CAD build for the part. Positions are in the model's coordinates, mm. A direction names the side the tool comes from. Give positions to 0.01 mm unless a question says otherwise; leave off trailing zeros. Write each loop counter-clockwise with the first axis right and the second up, starting at its lowest first coordinate (ties: lowest second). Pieces come first, ordered by that corner, then holes. Notation, with made-up numbers: (-30, 8) - (16, 8) arc R29 ccw to (16, 35) - close; hole circle Ø6 at (-3, 13). An arc over 180 degrees is marked (long way). Put each result on its own line as item: value. Start each with the question number.
1. Mould opens along X. For faces 3 (the cylindrical face through (0.16, 21.937, 5.916)), 4 (the cylindrical face through (-10.28, -7.77, 0.85)), 5 (the flat face through (0, 0, -10)) say: +X half, -X half, draft (parallel to the pull), parting line (faces both ways), or undercut.
2. Tool access for faces 1 (the flat face through (-1, 1, 12)), 2 (the cylindrical face through (-0.618, 57.997, 5.916)): list every direction of +Z, -Z, +X, -X, +Y, -Y with a clear straight run to the whole face (end or side of a thin tool).
3. Cut at D-D on x = 33.5. List the corners of the cut face in (y, z), and give its area (3 significant figures).
4. Cut at B-B on z = 9.25. Give the number of separate pieces and of enclosed holes in the cut face, and give its area (3 significant figures).
5. Cut at A-A on y = -14. List the corners of the cut face in (x, z).
6. Drop flat-ended pins along their axis: pin 1 (10 mm diameter, centred on y = -51.5, z = -2.5, fed in from -X); pin 2 (3 mm diameter, centred on y = 54, z = 4.5, fed in from +X); pin 3 (3.5 mm diameter, centred on x = -12.12, y = 7, fed in from -Z); pin 4 (5 mm diameter, centred on x = 60, z = 6, fed in from -Y). Give the stop position or say it passes through.
7. Wall check: line 1 (Y direction, x = 0, z = -1.75); line 2 (Y direction, x = 0, z = 6.5); line 3 (Y direction, x = 25, z = 1.25). Give the ranges that are in metal, low to high.
8. Cut at C-C on y = 7. List the corners of the cut face in (x, z), and give its area (3 significant figures).
from build123d import *

# Parameters (mm, degrees)
SKETCH1_R               = 85
SKETCH1_R_2             = 2
BOSS_EXTRUDE1_DEPTH     = 12
SKETCH3_R               = 22
BOSS_EXTRUDE2_DEPTH     = 10
CUT_EXTRUDE1_DEPTH      = 123.204746225
CUT_EXTRUDE1_DEPTH_BACK = 123.204746225
SKETCH5_R               = 2


with BuildPart() as part:
    # Sketch1 → Boss-Extrude1 (new body)
    with BuildSketch(Plane.XY):
        Circle(SKETCH1_R)
        with Locations((0, 14)):
            Circle(SKETCH1_R_2, mode=Mode.SUBTRACT)
        with Locations((12.124355653, 7)):
            Circle(SKETCH1_R_2, mode=Mode.SUBTRACT)
        with Locations((12.124355653, -7)):
            Circle(SKETCH1_R_2, mode=Mode.SUBTRACT)
        with Locations((0, -14)):
            Circle(SKETCH1_R_2, mode=Mode.SUBTRACT)
        with Locations((-12.124355653, -7)):
            Circle(SKETCH1_R_2, mode=Mode.SUBTRACT)
        with Locations((-12.124355653, 7)):
            Circle(SKETCH1_R_2, mode=Mode.SUBTRACT)
        with BuildLine():
            Line((-16.104768385, 19.179115852), (-39.269994022, 34.182407181))
            ThreePointArc((-39.269994022, 34.182407181), (-41.530272968, 37.914054118), (-40.000243417, 41.999768173))
            ThreePointArc((-40.000243417, 41.999768173), (0, 58), (40.000243417, 41.999768173))
            ThreePointArc((40.000243417, 41.999768173), (41.530272968, 37.914054118), (39.269994022, 34.182407181))
            Line((39.269994022, 34.182407181), (16.104768385, 19.179115852))
            ThreePointArc((16.104768385, 19.179115852), (13.523321314, 18.377673488), (10.90195317, 19.036921468))
            ThreePointArc((10.90195317, 19.036921468), (0, 21.937569645), (-10.90195317, 19.036921468))
            ThreePointArc((-10.90195317, 19.036921468), (-13.523321314, 18.377673488), (-16.104768385, 19.179115852))
        make_face(mode=Mode.SUBTRACT)
        with BuildLine():
            Line((8.557217358, -23.53669647), (9.96783597, -51.100016021))
            ThreePointArc((9.96783597, -51.100016021), (12.069397543, -54.923298475), (16.372744483, -55.641111043))
            ThreePointArc((16.372744483, -55.641111043), (50.229473419, -29), (56.372987899, 13.64134287))
            ThreePointArc((56.372987899, 13.64134287), (53.59967051, 17.009244357), (49.237829993, 16.917608839))
            Line((49.237829993, 16.917608839), (24.661985743, 4.357580618))
            ThreePointArc((24.661985743, 4.357580618), (22.67719276, 2.522703057), (21.937434187, -0.077092338))
            ThreePointArc((21.937434187, -0.077092338), (18.99849261, -10.968784822), (11.035481016, -18.95982913))
            ThreePointArc((11.035481016, -18.95982913), (9.153871447, -20.900376546), (8.557217358, -23.53669647))
        make_face(mode=Mode.SUBTRACT)
        with BuildLine():
            Line((-24.661985743, 4.357580618), (-49.237829993, 16.917608839))
            ThreePointArc((-49.237829993, 16.917608839), (-53.59967051, 17.009244357), (-56.372987899, 13.64134287))
            ThreePointArc((-56.372987899, 13.64134287), (-50.229473419, -29), (-16.372744483, -55.641111043))
            ThreePointArc((-16.372744483, -55.641111043), (-12.069397543, -54.923298475), (-9.96783597, -51.100016021))
            Line((-9.96783597, -51.100016021), (-8.557217358, -23.53669647))
            ThreePointArc((-8.557217358, -23.53669647), (-9.153871447, -20.900376546), (-11.035481016, -18.95982913))
            ThreePointArc((-11.035481016, -18.95982913), (-18.99849261, -10.968784822), (-21.937434187, -0.077092338))
            ThreePointArc((-21.937434187, -0.077092338), (-22.67719276, 2.522703057), (-24.661985743, 4.357580618))
        make_face(mode=Mode.SUBTRACT)
    extrude(amount=BOSS_EXTRUDE1_DEPTH)

    # Sketch3 → Boss-Extrude2 (add)
    with BuildSketch(Plane(origin=(0, 0, 0), x_dir=(-1, 0, 0), z_dir=(0, 0, -1))):
        with Locations(Location((0, 0, 0), (0, 0, 178.347435868))):
            Circle(SKETCH3_R)
    extrude(amount=BOSS_EXTRUDE2_DEPTH)

    # Sketch5 → Cut-Extrude1 (cut, two sides: drawn at the far end of the back side and taken through both)
    with BuildSketch(Plane.XY.offset(12).offset(-CUT_EXTRUDE1_DEPTH_BACK)):
        with Locations((0, 14)):
            Circle(SKETCH5_R)
        with Locations((12.124355653, 7)):
            Circle(SKETCH5_R)
        with Locations((12.124355653, -7)):
            Circle(SKETCH5_R)
        with Locations((0, -14)):
            Circle(SKETCH5_R)
        with Locations((-12.124355653, -7)):
            Circle(SKETCH5_R)
        with Locations((-12.124355653, 7)):
            Circle(SKETCH5_R)
    extrude(amount=CUT_EXTRUDE1_DEPTH + CUT_EXTRUDE1_DEPTH_BACK, mode=Mode.SUBTRACT)


solid = part.part
Report:
1. face 3: undercut
1. face 4: undercut
1. face 5: draft
2. face 1: +Z, +X, -X, +Y, -Y
2. face 2: +Z, -Z
3. outline: (-78.12, 0) - (-47.35, 0) - (-47.35, 12) - (-78.12, 12) - close; (8.87, 0) - (30.45, 0) - (30.45, 12) - (8.87, 12) - close; (47.35, 0) - (78.12, 0) - (78.12, 12) - (47.35, 12) - close
3. area: 997 mm²
4. separate pieces: 1
4. enclosed holes: 9
4. area: 15,700 mm²
5. outline: (-83.84, 0) - (-56.28, 0) - (-56.28, 12) - (-83.84, 12) - close; (-16.97, -10) - (-2, -10) - (-2, 12) - (-16.89, 12) - (-16.89, 0) - (-16.97, 0) - close; (2, -10) - (16.97, -10) - (16.97, 0) - (16.89, 0) - (16.89, 12) - (2, 12) - close; (56.28, 0) - (83.84, 0) - (83.84, 12) - (56.28, 12) - close
6. pin 1: stops at x = -70.71
6. pin 2: stops at x = 66.85
6. pin 3: passes through
6. pin 4: stops at y = -62.6
7. line 1: y = -22 to -16, -12 to 12, 16 to 22
7. line 2: y = -85 to -16, -12 to 12, 16 to 21.94, 58 to 85
7. line 3: y = -81.24 to -52.34, 4.53 to 24.94, 52.34 to 81.24
8. outline: (-84.71, 0) - (-57.58, 0) - (-57.58, 12) - (-84.71, 12) - close; (-29.83, 0) - (-20.86, 0) - (-20.86, -10) - (-14.12, -10) - (-14.12, 12) - (-29.83, 12) - close; (-10.12, -10) - (10.12, -10) - (10.12, 12) - (-10.12, 12) - close; (14.12, -10) - (20.86, -10) - (20.86, 0) - (29.83, 0) - (29.83, 12) - (14.12, 12) - close; (57.58, 0) - (84.71, 0) - (84.71, 12) - (57.58, 12) - close
8. area: 1,610 mm²
